Input: part model. Units: mm. Frame: model coordinates. Face numbers are marked on the shaded views. A direction names the side the tool comes from. Round coordinates to 2 decimals unless told otherwise and drop trailing zeros. Order: outer loops, then holes, each group sorted by start corner. A loop starts at its lowest first (then second) coordinate and runs counter-clockwise, first axis right, second up.
Item 1: Mould query, pull axis Z, two halves, no side actions, for the marked faces 1, 2 and 3. Classes: released by +Z, released by -Z, zero draft, split by the parting line, or undercut.
Item 2: Reachability of the marked faces 4, 5, 6, 7 and 8 from +Z, -Z, +X, -X, +Y, -Y: full face, straight path, thin tool, end or side. Return the list, or none.
Item 3: Cut plane C-C on x = 2.75. Output: boundary loops of the cut face in (y, z).
Item 4: Line query: L1, parallel to Y at x = 4.4, z = 0; L2, parallel to X at y = 0, z = -0.75; L3, parallel to Y at x = 3.5, z = 1. Output: solid intervals per line, ascending.
Item 5: First-contact query: pin 1 (1 mm diameter, centred on x = -3.5, y = 2.5, fed in from -Z); pin 2 (4 mm diameter, centred on x = -3, y = 1, fed in from +Z); pin 3 (1.8 mm diameter, centred on x = -5, y = -1, fed in from -Z). Flat tips, straight axial feed; report the tip coordinate or a pass-through.
Item 6: Cut plane B-B on y = 0. Output: boundary loops of the cut face in (x, z).
Item 7: Cut plane D-D on x = -0.75. Output: boundary loops of the cut face in (y, z).
Item 8: Cut plane A-A on z = 0. Output: boundary loops of the cut face in (x, y), then the cut area to 3 significant figures.
```python
from build123d import *

# Parameters (mm, degrees)
BOSS_EXTRUDE1_DEPTH = 7
SKETCH5_R           = 3.5
BOSS_EXTRUDE2_DEPTH = 6
FILLET1_R           = 0.5
CUT_EXTRUDE1_DEPTH  = 5


with BuildPart() as part:
    # Sketch1 → Boss-Extrude1 (new body)
    with BuildSketch(Plane(origin=(0, 0, 0), x_dir=(0, 0, -1), z_dir=(1, 0, 0))):
        with BuildLine():
            Line((-1.9, 1.84729532), (-1.9, -1.84729532))
            ThreePointArc((-1.9, -1.84729532), (0, -2.65), (1.9, -1.84729532))
            Line((1.9, -1.84729532), (1.9, 1.84729532))
            ThreePointArc((1.9, 1.84729532), (0, 2.65), (-1.9, 1.84729532))
        make_face()
    extrude(amount=-BOSS_EXTRUDE1_DEPTH)

    # Sketch5 → Boss-Extrude2 (add)
    with BuildSketch(Plane(origin=(0, 0, 0), x_dir=(0, 0, -1), z_dir=(1, 0, 0))):
        Circle(SKETCH5_R)
    extrude(amount=BOSS_EXTRUDE2_DEPTH)

    # Fillet1
    fillet1_edges = [part.edges().sort_by_distance(p)[0] for p in [
        (0, 0, -1.9),
        (0, -2.65, 0),
        (0, 0, 1.9),
        (0, 2.65, 0),
    ]]
    fillet(fillet1_edges, radius=FILLET1_R)

    # Sketch7 → Cut-Extrude1 (cut)
    with BuildSketch(Plane(origin=(6, 0, 0), x_dir=(0, 0, -1), z_dir=(1, 0, 0))):
        with BuildLine():
            Line((-1.316244658, 1.7), (1.316244658, 1.7))
            ThreePointArc((1.316244658, 1.7), (0, -2.15), (-1.316244658, 1.7))
        make_face()
    extrude(amount=-CUT_EXTRUDE1_DEPTH, mode=Mode.SUBTRACT)


solid = part.part
```
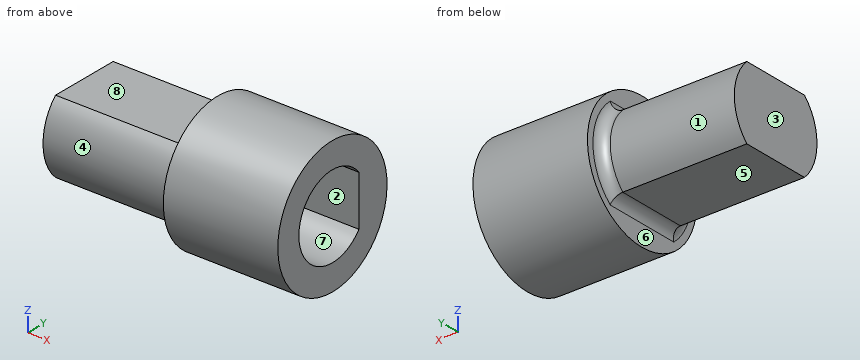
From the geometry:
1. face 1: split by the parting line
1. face 2: undercut
1. face 3: zero draft
2. face 4: -X, -Y
2. face 5: -Z, -X, +Y, -Y
2. face 6: -X
2. face 7: +X
2. face 8: +Z, -X, +Y, -Y
3. outline: circle Ø7 at (0, 0); hole (1.7, -1.32) - (1.7, 1.32) arc R2.15 ccw (long way) to start
4. L1: y = -3.5 to -2.15, 1.7 to 3.5
4. L2: x = -7 to 1
4. L3: y = -3.35 to -1.9, 1.7 to 3.35
5. pin 1: stops at z = -1.74
5. pin 2: stops at z = 1.9
5. pin 3: stops at z = -1.9
6. outline: (-7, -1.9) - (-0.5, -1.9) arc R0.5 cw to (0, -2.4) - (0, -3.5) - (6, -3.5) - (6, -2.15) - (1, -2.15) - (1, 2.15) - (6, 2.15) - (6, 3.5) - (0, 3.5) - (0, 2.4) arc R0.5 cw to (-0.5, 1.9) - (-7, 1.9) - close
7. outline: (-1.85, -1.9) - (1.85, -1.9) arc R2.65 ccw to (1.85, 1.9) - (-1.85, 1.9) arc R2.65 ccw to start
8. outline: (-7, -2.65) - (-0.5, -2.65) arc R0.5 cw to (0, -3.15) - (0, -3.5) - (6, -3.5) - (6, -2.15) - (1, -2.15) - (1, 1.7) - (6, 1.7) - (6, 3.5) - (0, 3.5) - (0, 3.15) arc R0.5 cw to (-0.5, 2.65) - (-7, 2.65) - close
8. area: 60.0 mm2
